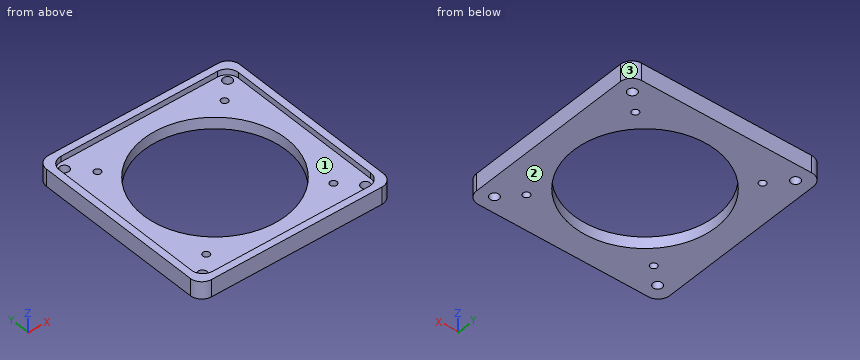
from build123d import *

# Parameters (mm, degrees)
EXTRUDE002_DEPTH = 9
SKETCH009_R      = 1.5
SKETCH009_R_2    = 31
SKETCH009_R_3    = 2
EXTRUDE001_DEPTH = 7.5


with BuildPart() as extrude002:
    # Sketch010 → Extrude002 (new body)
    with BuildSketch(Plane.XY):
        with BuildLine():
            Line((-34, 39), (34, 39))
            ThreePointArc((39, 34), (37.535534, 37.535534), (34, 39))
            Line((39, 34), (39, -34))
            ThreePointArc((34, -39), (37.535534, -37.535534), (39, -34))
            Line((34, -39), (-34, -39))
            ThreePointArc((-39, -34), (-37.535534, -37.535534), (-34, -39))
            Line((-39, -34), (-39, 34))
            ThreePointArc((-34, 39), (-37.535534, 37.535534), (-39, 34))
        make_face()
    extrude(amount=EXTRUDE002_DEPTH)


with BuildPart() as extrude002_1:
    # Extrude002 placement: moved
    add(extrude002.part.moved(Location((0, 0, 5))))


with BuildPart() as frontplate:
    # Sketch009 → Extrude001 (new body)
    with BuildSketch(Plane.XY):
        with BuildLine():
            Line((-37, 42), (37, 42))
            ThreePointArc((42, 37), (40.535534, 40.535534), (37, 42))
            Line((42, 37), (42, -37.141721))
            ThreePointArc((37.172983, -42), (40.548854, -40.527031), (42, -37.141721))
            Line((37.172983, -42), (-37, -42))
            ThreePointArc((-42, -37), (-40.535534, -40.535534), (-37, -42))
            Line((-42, -37), (-42, 37))
            ThreePointArc((-37, 42), (-40.535534, 40.535534), (-42, 37))
        make_face()
        with Locations((-28, 27.370892)):
            Circle(SKETCH009_R, mode=Mode.SUBTRACT)
        with Locations((28, 28.147012)):
            Circle(SKETCH009_R, mode=Mode.SUBTRACT)
        with Locations((28, -27.852988)):
            Circle(SKETCH009_R, mode=Mode.SUBTRACT)
        with Locations((-28, -28.629108)):
            Circle(SKETCH009_R, mode=Mode.SUBTRACT)
        Circle(SKETCH009_R_2, mode=Mode.SUBTRACT)
        with Locations((35.5, -35.5)):
            Circle(SKETCH009_R_3, mode=Mode.SUBTRACT)
        with Locations((-35.5, -35.5)):
            Circle(SKETCH009_R_3, mode=Mode.SUBTRACT)
        with Locations((-35.5, 35.5)):
            Circle(SKETCH009_R_3, mode=Mode.SUBTRACT)
        with Locations((35.5, 35.5)):
            Circle(SKETCH009_R_3, mode=Mode.SUBTRACT)
    extrude(amount=EXTRUDE001_DEPTH)

    # Cut028: cut Extrude002
    add(extrude002_1.part, mode=Mode.SUBTRACT)


with BuildPart() as frontplate_1:
    # Cut028 placement: moved
    add(frontplate.part.moved(Location((0, 0, 67))))


solid = frontplate_1.part
Geometry check sheet. Reference: the model listing, model coordinates, mm. Face numbers are marked on the shaded views. Round coordinates to 2 decimals unless told otherwise and drop trailing zeros. Loops run counter-clockwise (first coordinate to the right, second up) from the corner with the lowest first, then second, coordinate; pieces in that order, holes last.
Item 1: Cross-section at A-A on z = 73.5. Record the boundary of the cut face in (x, y), then the cut area to 3 significant figures.
Item 2: Cross-section at D-D on x = 35.5. Record the boundary of the cut face in (y, z), then the cut area to 3 significant figures.
Item 3: Mould release check, pull along Y, two halves, no side actions. Record for the marked faces 1, 2 and 3: pulls with the +Y half, pulls with the -Y half, needs draft (parallel to the pull), parting line crosses it, or undercut.
Item 4: Cross-section at B-B on y = 0. Record the boundary of the cut face in (x, z).
Item 5: Gauge pin test, flat ends, axial feed: pin 1 (2.5 mm diameter, centred on x = -28, y = 27.37, fed in from +Z); pin 2 (5 mm diameter, centred on x = 28, y = -27.85, fed in from +Z). Record the tip position at first contact, or that the pin passes through.
Item 6: Thickness scan on line 1 (Y direction, x = 35.5, z = 69.7); line 2 (Y direction, x = -6, z = 73); line 3 (Y direction, x = -28, z = 68.65). Record the ranges inside material, lowest first.
Answer sheet:
1. outline: (-42, -37) arc R5 ccw to (-37, -42) - (37.17, -42) arc R5 ccw to (42, -37.14) - (42, 37) arc R5 ccw to (37, 42) - (-37, 42) arc R5 ccw to (-42, 37) - close; hole (-39, -34) arc R5 ccw to (-34, -39) - (34, -39) arc R5 ccw to (39, -34) - (39, 34) arc R5 ccw to (34, 39) - (-34, 39) arc R5 ccw to (-39, 34) - close
1. area: 972 mm2
2. outline: (-42, 67) - (-37.5, 67) - (-37.5, 72) - (-38.77, 72) - (-38.77, 74.5) - (-42, 74.5) - close; (-33.5, 67) - (33.5, 67) - (33.5, 72) - (-33.5, 72) - close; (37.5, 67) - (42, 67) - (42, 74.5) - (38.77, 74.5) - (38.77, 72) - (37.5, 72) - close
2. area: 396 mm2
3. face 1: undercut
3. face 2: needs draft
3. face 3: pulls with the +Y half
4. outline: (-42, 67) - (-31, 67) - (-31, 72) - (-39, 72) - (-39, 74.5) - (-42, 74.5) - close; (31, 67) - (42, 67) - (42, 74.5) - (39, 74.5) - (39, 72) - (31, 72) - close
5. pin 1: passes through
5. pin 2: stops at z = 72
6. line 1: y = -42 to -37.5, -33.5 to 33.5, 37.5 to 42
6. line 2: y = -42 to -39, 39 to 42
6. line 3: y = -42 to -30.13, -27.13 to -13.3, 13.3 to 25.87, 28.87 to 42
